Autodesk Inventor part; units mm, degrees
ref_plane "YZ Plane" through (0, 0, 0) normal (1, 0, 0) x (0, 1, 0)
ref_plane "XZ Plane" through (0, 0, 0) normal (0, 1, 0) x (-1, 0, 0)
ref_plane "XY Plane" through (0, 0, 0) normal (0, 0, 1) x (1, 0, 0)
sketch "Sketch1" plane through (0, 0, 0) normal (0, 1, 0) x (-1, 0, 0)
  line L0 (0, 0) -> (22.7, 0)
  line L1 (22.7, 0) -> (22.7, 108)
  line L2 (22.7, 108) -> (10, 108)
  line L3 (10, 108) -> (10, 17.8)
  line L4 (10, 17.8) -> (0, 17.8)
  line L5 (0, 17.8) -> (0, 0)
  dimension "d0" = 22.7
  dimension "d1" = 108
  dimension "d2" = 12.7
  dimension "d3" = 90.2
extrude "Extrusion1" add sketch "Sketch1" along normal blind 12.5
sketch "Sketch2" plane through (0, 12.5, 0) normal (0, 1, 0) x (1, 0, 0)
  line L0 (0, -17.8) -> (0, 0)
  line L1 (-22.7, 0) -> (-22.7, -108)
  line L2 (-22.7, 0) -> (-22.7, -108)
  line L3 (0, -15.3) -> (-22.7, -15.3)
  line L4 (-22.7, -15.3) -> (-22.7, -2.5)
  line L5 (-22.7, -2.5) -> (0, -2.5)
  line L6 (0, -2.5) -> (0, -15.3)
  dimension "d6" = 12.8
extrude "Extrusion2" cut sketch "Sketch2" against normal blind 3.5
sketch "Sketch3" plane through (0, 9, 0) normal (0, 1, 0) x (1, 0, 0)
  line L0 (-30, -8.9) -> (0, -8.9) construction
  line L1 (0, -17.8) -> (0, 0)
  arc A0 (-4, -10.9) -> (-4, -6.9) centre (-4, -8.9) ccw
  arc A1 (-19, -6.9) -> (-19, -10.9) centre (-19, -8.9) ccw
  line L2 (-19, -10.9) -> (-4, -10.9)
  line L3 (-4, -6.9) -> (-19, -6.9)
  dimension "d9" = 4
  dimension "d10" = 4
  dimension "d26" = 15
  dimension "d27" = 4
extrude "Extrusion3" cut sketch "Sketch3" against normal through all
sketch "Sketch4" plane through (0, 12.5, 0) normal (0, 1, 0) x (1, 0, 0)
  line L0 (-22.7, -108) -> (-10, -108)
  line L1 (-16.35, -108) -> (-16.35, -15.5103) construction
  circle A0 centre (-16.35, -101.5) radius 5.5
  circle A1 centre (-16.35, -89) radius 5.5
  circle A2 centre (-16.35, -76.5) radius 5.5
  circle A3 centre (-16.35, -76.5) radius 3.25
  circle A4 centre (-16.35, -89) radius 3.25
  circle A5 centre (-16.35, -101.5) radius 3.25
  point P0 (0, 0)
  dimension "d13" = 11
  dimension "d14" = 11
  dimension "d15" = 11
  dimension "d16" = 12.5
  dimension "d17" = 12.5
  dimension "d18" = 6.5
  dimension "d19" = 6.5
  dimension "d20" = 6.5
  dimension "d25" = 6.5
extrude "Extrusion4" cut sketch "Sketch4" against normal through all contours A3 | A4 | A5
extrude "Extrusion5" cut sketch "Sketch4" against normal blind 6
properties part number "HeadbarHolder" material "Aluminum 6061"
Model file for the job. Use its own axes, mm. A direction names the side the tool comes from. Coordinates: 2 decimals unless noted, no trailing zeros. Order: outer loops, then holes, each group sorted by start corner. A loop starts at its lowest first (then second) coordinate and runs counter-clockwise, first axis right, second up. Notation, with made-up numbers: (-28, 80) -> (14, 80) arc R24 ccw to (14, 95) -> close; hole circle Ø10 at (-23.5, 15.5). An arc over 180 degrees is marked (long way). Answer as a JSON object with one key per item and string values. Group by question number.
1) Cut at A-A, the plane y = 11. Write the cut outline in (x, z), then the cut area to 3 significant figures.
2) Drill centre lines: L1, parallel to Z at x = -16.35, y = 10.35; L2, parallel to X at y = 8.55, z = 101.5; L3, parallel to Z at x = -18, y = 3. Where is each one in solid material? Low to high.
3) Pull direction X, two halves, no side cores. Call faces 1 (the face through (-16, 0, 43)), 2 (the face through (-14, 6.5, 79)), 3 (the face through (-10, 6, 64)): +X half, -X half, draft (parallel to the pull), parting line (faces both ways), or undercut.
4) Cut at B-B, the plane z = 89. Write the cut outline in (x, y).
5) Cut at C-C, the plane y = 4.25. Write the cut outline in (x, z).
6) Which spindle directions (+Z, -Z, +X, -X, +Y, -Y) get a long thin tool onto all of the face, cutting with end or side? Do faces 4 (the face through (-17.066, 9.542, 71.047)), 5 (the face through (-21, 4.6, 8.9)), 6 (the face through (-11, 11, 15.3)). Say none if no direction does.
7) Flat gauge pins, fed straight in: pin 1 (9 mm diameter, centred on x = -15.5, z = 76.5, fed in from +Y); pin 2 (6 mm diameter, centred on y = 3, z = 62.5, fed in from +X); pin 3 (5 mm diameter, centred on x = -5, y = 9, fed in from +Z). Where does each tip first touch, or does it go through?
8) Cut at D-D, the plane z = 8.9. Write the cut outline in (x, y), then the cut area to 3 significant figures.
Check values:
{
 "1": {"outline": "(-22.7, 0) -> (0, 0) -> (0, 2.5) -> (-22.7, 2.5) -> close; (-22.7, 15.3) -> (0, 15.3) -> (0, 17.8) -> (-10, 17.8) -> (-10, 108) -> (-22.7, 108) -> close; hole circle Ø11 at (-16.35, 76.5); hole circle Ø11 at (-16.35, 89); hole circle Ø11 at (-16.35, 101.5)", "area": "974 mm²"},
 "2": {"L1": "z = 0 to 2.5, 15.3 to 71, 82 to 83.5, 94.5 to 96, 107 to 108", "L2": "x = -22.7 to -21.85, -10.85 to -10", "L3": "z = 0 to 6.9, 10.9 to 73.7, 79.3 to 86.2, 91.8 to 98.7, 104.3 to 108"},
 "3": {"face 1": "draft", "face 2": "undercut", "face 3": "+X half"},
 "4": {"outline": "(-22.7, 0) -> (-19.6, 0) -> (-19.6, 6.5) -> (-21.85, 6.5) -> (-21.85, 12.5) -> (-22.7, 12.5) -> close; (-13.1, 0) -> (-10, 0) -> (-10, 12.5) -> (-10.85, 12.5) -> (-10.85, 6.5) -> (-13.1, 6.5) -> close"},
 "5": {"outline": "(-22.7, 0) -> (0, 0) -> (0, 17.8) -> (-10, 17.8) -> (-10, 108) -> (-22.7, 108) -> close; hole circle Ø6.5 at (-16.35, 76.5); hole circle Ø6.5 at (-16.35, 89); hole circle Ø6.5 at (-16.35, 101.5); hole (-19, 6.9) -> (-4, 6.9) arc R2 ccw to (-4, 10.9) -> (-19, 10.9) arc R2 ccw to start"},
 "6": {"face 4": "+Y", "face 5": "+Y, -Y", "face 6": "+X, -X, +Y"},
 "7": {"pin 1": "stops at y = 6.5", "pin 2": "stops at x = -10", "pin 3": "stops at z = 17.8"},
 "8": {"outline": "(-22.7, 0) -> (-21, 0) -> (-21, 9) -> (-22.7, 9) -> close; (-2, 0) -> (0, 0) -> (0, 9) -> (-2, 9) -> close", "area": "33.3 mm²"}
}
